Check sheet for the drawn part. Datum: minimum x, y, z corner. Units: mm. Give positions to 0.01 mm unless a question says otherwise; leave off trailing zeros. Write each loop counter-clockwise with the first axis right and the second up, starting at its lowest first coordinate (ties: lowest second). Pieces come first, ordered by that corner, then holes.
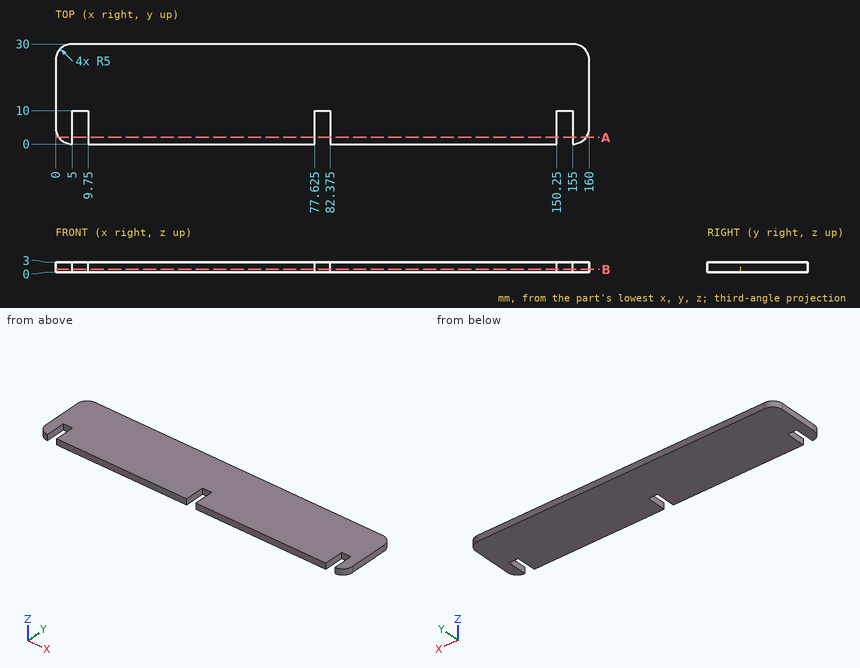
1) Sectioned sample at A-A on y = 2. Record the boundary of the cut face in (x, z) (3 decimals).
2) Scan lines: L1, parallel to X at y = 7, z = 0.9 (3 decimals); L2, parallel to X at y = 25.5, z = 1.5; L3, parallel to X at y = 26, z = 2. Record each from-to range of solid material in increasing order.
3) Gauge pin test, flat end, axial feed: pin 1 (0.9 mm diameter, centred on x = 7.5, z = 2, fed in from -Y). Record the tip position at first contact, or that the pin passes through.
4) Sectioned sample at B-B on z = 0.8. Record the boundary of the cut face in (x, y) (3 decimals), then the cut area to 3 significant figures.
Answers below:
1. outline: (1, 0) - (5, 0) - (5, 3) - (1, 3) - close; (9.75, 0) - (77.625, 0) - (77.625, 3) - (9.75, 3) - close; (82.375, 0) - (150.25, 0) - (150.25, 3) - (82.375, 3) - close; (155, 0) - (159, 0) - (159, 3) - (155, 3) - close
2. L1: x = 0 to 5, 9.75 to 77.625, 82.375 to 150.25, 155 to 160
2. L2: x = 0.03 to 159.97
2. L3: x = 0.1 to 159.9
3. pin 1: stops at y = 10
4. outline: (0, 5) arc R5 ccw to (5, 0) - (5, 10) - (9.75, 10) - (9.75, 0) - (77.625, 0) - (77.625, 10) - (82.375, 10) - (82.375, 0) - (150.25, 0) - (150.25, 10) - (155, 10) - (155, 0) arc R5 ccw to (160, 5) - (160, 25) arc R5 ccw to (155, 30) - (5, 30) arc R5 ccw to (0, 25) - close
4. area: 4,640 mm2
